Read the model definition and answer for the solid it produces. Units are mm, in the model's axes. A direction names the side the tool comes from. Give positions to 0.01 mm unless a question says otherwise; leave off trailing zeros. Write each loop counter-clockwise with the first axis right and the second up, starting at its lowest first coordinate (ties: lowest second). Pieces come first, ordered by that corner, then holes.
```python
from build123d import *

# Parameters (mm, degrees)
F0_W     = 6.75
F0_H     = 11.5
F0_W_2   = 11.5
F1_DEPTH = 5
F2_DEPTH = 20
F3_DEPTH = 25
F4_R     = 1.7
F5_DEPTH = 25.001
F6_W     = 5.5
F6_H     = 3
F7_DEPTH = 11.501
F8_R     = 1.7
F9_DEPTH = 45.001
F10_R    = 2


with BuildPart() as f1:
    # F0 (on Top) → F1 (new body)
    with BuildSketch(Plane.XY):
        with Locations((-9.125, 0)):
            Rectangle(F0_W, F0_H)
        with Locations((9.125, 0)):
            Rectangle(F0_W, F0_H)
        Rectangle(F0_W_2, F0_H)
    extrude(amount=-F1_DEPTH)

    # F0 (on Top) → F2 (join)
    with BuildSketch(Plane.XY):
        with Locations((9.125, 0)):
            Rectangle(F0_W, F0_H)
        with Locations((-9.125, 0)):
            Rectangle(F0_W, F0_H)
    extrude(amount=-F2_DEPTH)

    # F0 (on Top) → F3 (join)
    with BuildSketch(Plane.XY):
        Rectangle(F0_W_2, F0_H)
    extrude(amount=F3_DEPTH)

    # F4 (on face) → F5 (cut, through all)
    with BuildSketch(Plane(origin=(-12.5, 0, 0), x_dir=(0, -1, 0), z_dir=(-1, 0, 0))):
        with Locations((0, -15)):
            Circle(F4_R)
    extrude(amount=-F5_DEPTH, mode=Mode.SUBTRACT)

    # F6 (on face) → F7 (cut, through all)
    with BuildSketch(Plane(origin=(0, 5.75, 0), x_dir=(-1, 0, 0), z_dir=(0, 1, 0))):
        with Locations((0, 19.5)):
            Rectangle(F6_W, F6_H)
    extrude(amount=-F7_DEPTH, mode=Mode.SUBTRACT)

    # F8 (on face) → F9 (cut, through all)
    with BuildSketch(Plane.XY.offset(25)):
        Circle(F8_R)
    extrude(amount=-F9_DEPTH, mode=Mode.SUBTRACT)

    # F10
    f10_edges = [f1.edges().sort_by_distance(p)[0] for p in [
        (-5.75, 0, -20),
        (-12.5, 0, -20),
        (-5.75, 0, -5),
        (5.75, 0, -5),
        (5.75, 0, -20),
        (12.5, 0, -20),
        (12.5, 0, 0),
        (-12.5, 0, 0),
        (-5.75, 0, 0),
        (-5.75, 0, 25),
        (5.75, 0, 25),
        (5.75, 0, 0),
    ]]
    fillet(f10_edges, radius=F10_R)


solid = f1.part
```
Item 1: Section D-D (y = -4.25) is taken. Write down the section's boundary in (x, z), and give its area (3 significant figures).
Result set:
outline: (-12.5, -18) arc R2 ccw to (-10.5, -20) - (-7.75, -20) arc R2 ccw to (-5.75, -18) - (-5.75, -7) arc R2 cw to (-3.75, -5) - (3.75, -5) arc R2 cw to (5.75, -7) - (5.75, -18) arc R2 ccw to (7.75, -20) - (10.5, -20) arc R2 ccw to (12.5, -18) - (12.5, -2) arc R2 ccw to (10.5, 0) - (7.75, 0) arc R2 cw to (5.75, 2) - (5.75, 23) arc R2 ccw to (3.75, 25) - (-3.75, 25) arc R2 ccw to (-5.75, 23) - (-5.75, 2) arc R2 cw to (-7.75, 0) - (-10.5, 0) arc R2 ccw to (-12.5, -2) - close; hole (-2.75, 18) - (2.75, 18) - (2.75, 21) - (-2.75, 21) - close
area: 595 mm2
Item 2: Determine the mould class of faces 1 (the flat face through (1.3, 1.4, 21)), 2 (the cylindrical face through (6.35, 0.08, -19.43)), 3 (the flat face through (-2, 0, 25)) for opening direction Z: pulls with the +Z half, pulls with the -Z half, needs draft (parallel to the pull), parting line crosses it, or undercut.
Result set:
face 1: undercut
face 2: pulls with the -Z half
face 3: pulls with the +Z half
Item 3: Each of these flat-tipped pins is pushed along its axis until it touches: pin 1 Ø3 at (y, z) = (2, 16.5) entering from -X; pin 2 Ø2.5 at (y, z) = (1, 20) entering from +X; pin 3 Ø2 at (x, y) = (0, 0) entering from -Z; pin 4 Ø1.4 at (x, y) = (-9.5, 1) entering from +Z. Where does it stop, or does it pass through?
Result set:
pin 1: stops at x = -5.75
pin 2: stops at x = 5.75
pin 3: passes through
pin 4: stops at z = 0
Item 4: Section B-B (z = -10) is taken. Write down the section's boundary in (x, y).
Result set:
outline: (-12.5, -5.75) - (-5.75, -5.75) - (-5.75, 5.75) - (-12.5, 5.75) - close; (5.75, -5.75) - (12.5, -5.75) - (12.5, 5.75) - (5.75, 5.75) - close
Item 5: Find the intervals of material crossed by line 1 along Z through (x, y) = (10.5, 0); line 2 along Y through (x, z) = (0, 3); line 3 along Z through (x, y) = (-2.25, 1.5), in increasing order.
Result set:
line 1: z = -20 to -16.7, -13.3 to 0
line 2: y = -5.75 to -1.7, 1.7 to 5.75
line 3: z = -5 to 18, 21 to 25
Item 6: Section A-A (x = 0) is taken. Write down the section's boundary in (y, z).
Result set:
outline: (-5.75, -5) - (-1.7, -5) - (-1.7, 18) - (-5.75, 18) - close; (-5.75, 21) - (-1.7, 21) - (-1.7, 25) - (-5.75, 25) - close; (1.7, -5) - (5.75, -5) - (5.75, 18) - (1.7, 18) - close; (1.7, 21) - (5.75, 21) - (5.75, 25) - (1.7, 25) - close
Item 7: Section C-C (z = -15) is taken. Write down the section's boundary in (x, y), and give its area (3 significant figures).
Result set:
outline: (-12.5, -5.75) - (-5.75, -5.75) - (-5.75, -1.7) - (-12.5, -1.7) - close; (-12.5, 1.7) - (-5.75, 1.7) - (-5.75, 5.75) - (-12.5, 5.75) - close; (5.75, -5.75) - (12.5, -5.75) - (12.5, -1.7) - (5.75, -1.7) - close; (5.75, 1.7) - (12.5, 1.7) - (12.5, 5.75) - (5.75, 5.75) - close
area: 109 mm2
Item 8: Which of the six approach directions +Z, -Z, +X, -X, +Y, -Y give full straight-line access (tool end or side, diameter ignored) to faces 4 (the flat face through (5.75, 0, -12)), 5 (the flat face through (5.75, 0, 12)), 6 (the flat face through (1.3, 1.4, 18))?
Result set:
face 4: -Z, +Y, -Y
face 5: +Z, +X, +Y, -Y
face 6: +Y, -Y
